from build123d import *

# Parameters (mm, degrees)
SKETCH1_W           = 19
SKETCH1_H           = 90
BOSS_EXTRUDE2_DEPTH = 19
SKETCH2_W           = 16.74
SKETCH2_H           = 87.18
CUT_EXTRUDE1_DEPTH  = 17
SKETCH3_W           = 6
SKETCH3_H           = 6
BOSS_EXTRUDE4_DEPTH = 1
SKETCH5_W           = 6
SKETCH5_H           = 6
BOSS_EXTRUDE5_DEPTH = 1


with BuildPart() as part:
    # Sketch1 → Boss-Extrude2 (new body)
    with BuildSketch(Plane(origin=(0, 0, 0), x_dir=(1, 0, 0), z_dir=(0, 1, 0))):
        with Locations((-3.599862385, 31.801317605)):
            Rectangle(SKETCH1_W, SKETCH1_H)
    extrude(amount=BOSS_EXTRUDE2_DEPTH)

    # Sketch2 → Cut-Extrude1 (cut)
    with BuildSketch(Plane(origin=(0, 19, 0), x_dir=(1, 0, 0), z_dir=(0, 1, 0))):
        with Locations((-3.599862385, 31.801317605)):
            Rectangle(SKETCH2_W, SKETCH2_H)
    extrude(amount=-CUT_EXTRUDE1_DEPTH, mode=Mode.SUBTRACT)

    # Sketch3 → Boss-Extrude4 (add)
    with BuildSketch(Plane(origin=(0, 0, 11.788682395), x_dir=(-1, 0, 0), z_dir=(0, 0, -1))):
        with Locations((3.599862385, 10.5)):
            Rectangle(SKETCH3_W, SKETCH3_H)
    extrude(amount=BOSS_EXTRUDE4_DEPTH)

    # Sketch5 → Boss-Extrude5 (add)
    with BuildSketch(Plane.XY.offset(-75.391317605)):
        with Locations((-3.599862385, 10.5)):
            Rectangle(SKETCH5_W, SKETCH5_H)
    extrude(amount=BOSS_EXTRUDE5_DEPTH)


solid = part.part
Design review of the part built by this model. Coordinates are the model's own, in mm. A direction names the side the tool comes from. Round coordinates to 2 decimals unless told otherwise and drop trailing zeros. Loops run counter-clockwise (first coordinate to the right, second up) from the corner with the lowest first, then second, coordinate; pieces in that order, holes last. Notation, with made-up numbers: (-17, 22.5) - (25, 22.5) arc R13 ccw to (25, 40.5) - close; hole circle Ø7 at (14, 8). An arc over 180 degrees is marked (long way). One line per item, written item: value. Start each with the question number.
1) To check wall thickness, follow L1, parallel to Z at x = -8, y = 16.75; L2, parallel to X at y = 10, z = -47; L3, parallel to Y at x = -4.5, z = -54. State the ranges of each line that lie inside material, in increasing order. Write a range as from..to.
2) Consider section A-A on y = 11.5. Give the boundary of the cut face in (x, z), then the cut area to 3 significant figures.
3) For faces 1 (the flat face through (4.77, 11, -31)), 2 (the flat face through (-7, 11, -75.391)), 3 (the flat face through (-4, 9, 13.199)), list the 3-axis set-ups (+Z, -Z, +X, -X, +Y, -Y) from which the entire face can be reached by the end or side of a thin tool; tool diameter is ignored.
4) Insertion check: pin 1 Ø1.5 at (x, z) = (-8, -32) entering from +Y; pin 2 Ø0.5 at (x, z) = (-3.5, 11) entering from +Y. Each pin has a flat end and moves straight along its axis. Give the tip position at first contact, or say it passes through.
5) Draft analysis for pull direction X (two halves, no side actions). For faces 4 (the flat face through (-4, 0, -32)), 5 (the flat face through (-13.1, 9, -31)), 6 (the flat face through (-4, 2, -32)), state which applies: +X half, -X half, draft (parallel to the pull), parting line (faces both ways), or undercut.
6) Consider section B-B on z = -24. Give the boundary of the cut face in (x, y), then the cut area to 3 significant figures.
7) Consider section D-D on x = 2.5. Give the boundary of the cut face in (y, z), then the cut area to 3 significant figures.
8) Consider section C-C on x = -2.25. Give the boundary of the cut face in (y, z).
Reported:
1. L1: z = -76.8..-75.39, 11.79..13.2
1. L2: x = -13.1..-11.97, 4.77..5.9
1. L3: y = 0..2
2. outline: (-13.1, -76.8) - (5.9, -76.8) - (5.9, 13.2) - (-13.1, 13.2) - close; hole (-11.97, -75.39) - (-6.6, -75.39) - (-6.6, -74.39) - (-0.6, -74.39) - (-0.6, -75.39) - (4.77, -75.39) - (4.77, 11.79) - (-0.6, 11.79) - (-0.6, 10.79) - (-6.6, 10.79) - (-6.6, 11.79) - (-11.97, 11.79) - close
2. area: 263 mm^2
3. face 1: +Y
3. face 2: none
3. face 3: +Z, +X, -X, +Y, -Y
4. pin 1: stops at y = 2
4. pin 2: stops at y = 13.5
5. face 4: draft
5. face 5: -X half
5. face 6: undercut
6. outline: (-13.1, 0) - (5.9, 0) - (5.9, 19) - (4.77, 19) - (4.77, 2) - (-11.97, 2) - (-11.97, 19) - (-13.1, 19) - close
6. area: 76.4 mm^2
7. outline: (0, -76.8) - (19, -76.8) - (19, -75.39) - (2, -75.39) - (2, 11.79) - (19, 11.79) - (19, 13.2) - (0, 13.2) - close
7. area: 228 mm^2
8. outline: (0, -76.8) - (19, -76.8) - (19, -75.39) - (13.5, -75.39) - (13.5, -74.39) - (7.5, -74.39) - (7.5, -75.39) - (2, -75.39) - (2, 11.79) - (7.5, 11.79) - (7.5, 10.79) - (13.5, 10.79) - (13.5, 11.79) - (19, 11.79) - (19, 13.2) - (0, 13.2) - close
